```python
from build123d import *

# Parameters (mm, degrees)
F1_DEPTH = 42
F2_T     = -2.5


with BuildPart() as f1:
    # F0 (on Front) → F1 (new body)
    with BuildSketch(Plane.XZ):
        with BuildLine():
            Line((95, 0), (0, 0))
            Line((0, 0), (0, -70))
            ThreePointArc((0, -70), (5.857864, -84.142136), (20, -90))
            Line((20, -90), (75, -90))
            ThreePointArc((75, -90), (89.142136, -84.142136), (95, -70))
            Line((95, -70), (95, 0))
        make_face()
    extrude(amount=F1_DEPTH)

    # F2
    f2_openings = [f1.faces().sort_by_distance(p)[0] for p in [
        (47.5, -21, 0),
    ]]
    offset(amount=F2_T, openings=f2_openings)


solid = f1.part
```
The model under review builds one solid part; all positions refer to its coordinate system, in mm. A direction names the side the tool comes from. Coordinates: 2 decimals unless noted, no trailing zeros. Write each loop counter-clockwise with the first axis right and the second up, starting at its lowest first coordinate (ties: lowest second). Pieces come first, ordered by that corner, then holes. Notation, with made-up numbers: (58, 65.5) - (101, 65.5) arc R30 ccw to (101, 90.5) - close; hole circle Ø2 at (84.5, -1.5). An arc over 180 degrees is marked (long way). Answer in a Markdown table with one row per item. Add a question column.
Q1. For faces 1 (the face through (5.703, -20.706, -83.986)), 2 (the face through (2.5, -21, -35)), list the 3-axis set-ups (+Z, -Z, +X, -X, +Y, -Y) from which the entire face can be reached by the end or side of a thin tool; tool diameter is ignored.
Q2. To check wall thickness, follow line 1 along Y through (x, z) = (24.5, -52.5); line 2 along X through (y, z) = (-34, -55); line 3 along X through (y, z) = (-32, -76). State the ranges of each line that lie inside material, in increasing order. Write a range as from..to.
Q3. Consider section D-D on x = 26. Give the boundary of the cut face in (y, z).
Q4. Consider section C-C on x = 11. Give the boundary of the cut face in (y, z), then the cut area to 3 significant figures.
Q5. Clearance check with a flat-ended pin moving along its axis: pin 1 (4 mm diameter, centred on x = 65.5, y = -21, fed in from +Z). State where the tip first meets the part, or that it passes through.
Q6. Consider section A-A on y = -26.5. Give the boundary of the cut face in (x, z), then the cut area to 3 significant figures.
Q7. Consider section B-B on z = -45.5. Give the boundary of the cut face in (x, y), then the cut area to 3 significant figures.
Q8. Draft analysis for pull direction Y (two halves, no side actions). For faces 3 (the face through (47, 0, -44)), 4 (the face through (95, -21, -35)), 5 (the face through (92.5, -21, -35)), state which applies: +Y half, -Y half, draft (parallel to the pull), parting line (faces both ways), or undercut.
Answers below:
| question | item | result |
|---|---|---|
| 1 | face 1 | -Z, -X, +Y, -Y |
| 1 | face 2 | +Z |
| 2 | line 1 | -42..-39.5, -2.5..0 |
| 2 | line 2 | 0..2.5, 92.5..95 |
| 2 | line 3 | 0.92..3.56, 91.44..94.08 |
| 3 | outline | (-42, -90) - (0, -90) - (0, 0) - (-2.5, 0) - (-2.5, -87.5) - (-39.5, -87.5) - (-39.5, 0) - (-42, 0) - close |
| 4 | outline | (-42, -87.86) - (0, -87.86) - (0, 0) - (-2.5, 0) - (-2.5, -85.01) - (-39.5, -85.01) - (-39.5, 0) - (-42, 0) - close |
| 4 | area | 545 mm² |
| 5 | pin 1 | z = -87.5 |
| 6 | outline | (0, -70) arc R20 ccw to (20, -90) - (75, -90) arc R20 ccw to (95, -70) - (95, 0) - (92.5, 0) - (92.5, -70) arc R17.5 cw to (75, -87.5) - (20, -87.5) arc R17.5 cw to (2.5, -70) - (2.5, 0) - (0, 0) - close |
| 6 | area | 635 mm² |
| 7 | outline | (0, -42) - (95, -42) - (95, 0) - (0, 0) - close; hole (2.5, -39.5) - (92.5, -39.5) - (92.5, -2.5) - (2.5, -2.5) - close |
| 7 | area | 660 mm² |
| 8 | face 3 | +Y half |
| 8 | face 4 | draft |
| 8 | face 5 | undercut |
